Geometry: final body of the model. Coordinates: model frame, mm. A direction names the side the tool comes from. Round coordinates to 2 decimals unless told otherwise and drop trailing zeros. Loops run counter-clockwise (first coordinate to the right, second up) from the corner with the lowest first, then second, coordinate; pieces in that order, holes last. Notation, with made-up numbers: M 64,73 L 88,73 A9 cw 88,89 Z; hole C -2.75,25 d5. An arc over 180 degrees is marked long. Answer as a JSON object with one key per item and string values.
from build123d import *

# Parameters (mm, degrees)
EXTRUDE_1_DEPTH     = 45
SKETCH_2_R          = 43
CUT_EXTRUDE_1_DEPTH = 12.7
CUT_EXTRUDE_6_DEPTH = 33.5
SKETCH_6_W          = 0.8
SKETCH_6_H          = 3.2


with BuildPart() as part:
    # Эскиз1 → Бобышка-Вытянуть1 (new body)
    with BuildSketch(Plane.XY):
        with BuildLine():
            Line((-102, 0), (-102, -131))
            Line((-102, -131), (-55.5, -166.04026333))
            Line((-55.5, -166.04026333), (-55.5, -459.04026333))
            Line((-55.5, -459.04026333), (55.5, -459.04026333))
            Line((55.5, -459.04026333), (55.5, -166.04026333))
            Line((55.5, -166.04026333), (102, -131))
            Line((102, -131), (102, 0))
            ThreePointArc((102, 0), (0, 102), (-102, 0))
        make_face()
    extrude(amount=EXTRUDE_1_DEPTH)

    # Эскиз2 → Вырез-Вытянуть1 (cut)
    with BuildSketch(Plane.XY.offset(45)):
        Circle(SKETCH_2_R)
    extrude(amount=-CUT_EXTRUDE_1_DEPTH, mode=Mode.SUBTRACT)

    # Sketch 1 2 → Вырез-Вытянуть6 (cut)
    with BuildSketch(Plane(origin=(91.857329022, -138.643050794, 39.25), x_dir=(-0.7228095146046781, -0.6910473251499855, 0), z_dir=(0, 0, -1))):
        Polygon((0, 0), (45.212193782, 5.321669076), (51.742831193, -1.509132064), (53.321326579, 0), (39.707694274, 14.239347438), (-1.110524428, 9.43486807), align=None)
    cut_extrude_6 = extrude(amount=CUT_EXTRUDE_6_DEPTH, mode=Mode.SUBTRACT)

    # Зеркальное отражение1: Вырез-Вытянуть6 across plane
    add(cut_extrude_6.mirror(Plane(origin=(0, 0, 0), x_dir=(0, 0, 1), z_dir=(1, 0, 0))), mode=Mode.SUBTRACT)

    # Вырез-По траектории1: sweep along a curve in space
    with BuildLine() as sweep_1_path:
        Line((55.5, -295.44026333, 45), (55.5, -295.44026333, 0))
        Line((55.5, -295.44026333, 0), (-55.5, -295.44026333, 0))
        Line((-55.5, -295.44026333, 0), (-55.5, -295.44026333, 45))
        Line((-55.5, -295.44026333, 45), (55.5, -295.44026333, 45))
    # Эскиз6 → Вырез-По траектории1 (sweep, cut)
    with BuildSketch(Plane.XY.offset(45)):
        with Locations((55.1, -295.44026333)):
            Rectangle(SKETCH_6_W, SKETCH_6_H)
    sweep(path=sweep_1_path.line, transition=Transition.RIGHT, mode=Mode.SUBTRACT)


solid = part.part
1) Section query D-D (x = 30). Return the cut outline in (y, z), and give its area (3 significant figures).
Results:
{"outline": "M -459.04,0 L -297.04,0 L -297.04,0.8 L -293.84,0.8 L -293.84,0 L 97.49,0 L 97.49,45 L 30.81,45 L 30.81,32.3 L -30.81,32.3 L -30.81,45 L -293.84,45 L -293.84,44.2 L -297.04,44.2 L -297.04,45 L -459.04,45 Z", "area": "24,300 mm2"}
2) Section query B-B (z = 17). Return the cut outline in (x, y).
Results:
{"outline": "M -102,-131 L -91.86,-138.64 L -86.14,-131.06 L -53.32,-155.79 L -53.32,-175.49 L -55.5,-175.49 L -55.5,-293.84 L -54.7,-293.84 L -54.7,-297.04 L -55.5,-297.04 L -55.5,-459.04 L 55.5,-459.04 L 55.5,-297.04 L 54.7,-297.04 L 54.7,-293.84 L 55.5,-293.84 L 55.5,-175.49 L 53.32,-175.49 L 53.32,-155.79 L 86.14,-131.06 L 91.86,-138.64 L 102,-131 L 102,0 A102 ccw -102,0 Z"}
3) Pull-direction query (Y, two-part tool) for faces 1 (the flat face through (-94.58, -136.59, 22.18)), 2 (the flat face through (-55.5, -377, 22)), 3 (the cylindrical face through (2.243, 101.975, 22.185)), 4 (the cylindrical face through (-5.598, 42.634, 38.739)); classes: +Y half, -Y half, draft (parallel to the pull), parting line (faces both ways), or undercut.
Results:
{"face 1": "-Y half", "face 2": "draft", "face 3": "+Y half", "face 4": "undercut"}
4) Pin query (flat end, axial travel): P1, Ø4, axis at y = -310, z = 39.5, coming from the +X side; P2, Ø1.7, axis at x = 54.5, z = 28, coming from the +Y side; P3, Ø1, axis at y = -295.5, z = 31, coming from the -X side. Return the tip coordinate at first contact, or that it passes through.
Results:
{"P1": "x = 55.5", "P2": "y = 86.75", "P3": "x = -54.7"}
5) Section query C-C (y = -254). Return the cut outline in (x, z), and give its area (4 significant figures).
Results:
{"outline": "M -55.5,0 L 55.5,0 L 55.5,45 L -55.5,45 Z", "area": "4,995 mm2"}
6) Section query A-A (x = 0). Return the cut outline in (y, z), and give its area (3 significant figures).
Results:
{"outline": "M -459.04,0 L -297.04,0 L -297.04,0.8 L -293.84,0.8 L -293.84,0 L 102,0 L 102,45 L 43,45 L 43,32.3 L -43,32.3 L -43,45 L -293.84,45 L -293.84,44.2 L -297.04,44.2 L -297.04,45 L -459.04,45 Z", "area": "24,100 mm2"}
7) Reachability of faces 5 (the flat face through (-1, -93, 45)), 6 (the flat face through (-55.5, -229, 22)), 7 (the flat face through (55.5, -231, 22)) from +Z, -Z, +X, -X, +Y, -Y: full face, straight path, thin tool, end or side. Return the list, or none.
Results:
{"face 5": "+Z, +X, -X, +Y, -Y", "face 6": "+Z, -Z, -X, -Y", "face 7": "+Z, -Z, +X, -Y"}
8) Ray query, line 1 (Y direction, x = 0, z = 36.5); line 2 (X direction, y = -246, z = 20); line 3 (Y direction, x = -35.5, z = 43.5). Return the intervals inside material, ascending.
Results:
{"line 1": "-459.04 to -43, 43 to 102", "line 2": "-55.5 to 55.5", "line 3": "-459.04 to -24.26, 24.26 to 95.62"}
